```python
from build123d import *

# Parameters (mm, degrees)
SKETCH1_R           = 1.75
SKETCH1_W           = 15
SKETCH1_H           = 5
BOSS_EXTRUDE1_DEPTH = 5
FILLET1_R           = 5


with BuildPart() as part:
    # Sketch1 → Boss-Extrude1 (new body)
    with BuildSketch(Plane(origin=(0, 0, 0), x_dir=(1, 0, 0), z_dir=(0, 1, 0))):
        Polygon((65, 15), (65, 30), (60, 30), (60, 35), (50, 35), (50, 30), (0, 30), (0, 35), (-10, 35), (-10, 30), (-65, 30), (-65, 20), (-72.992352801, 20), (-72.992352801, 5), (-72.992352801, -5), (-72.992352801, -20), (-65, -20), (-65, -30), (-10, -30), (-10, -35), (0, -35), (0, -30), (50, -30), (50, -35), (60, -35), (60, -30), (65, -30), (65, -15), (85, -15), (85, -5), (65, -5), (65, 5), (85, 5), (85, 15), align=None)
        with Locations(Location((27, 20, 0), (0, 0, 270))):
            Circle(SKETCH1_R, mode=Mode.SUBTRACT)
        with Locations(Location((27, -20, 0), (0, 0, 270))):
            Circle(SKETCH1_R, mode=Mode.SUBTRACT)
        with Locations(Location((-31, 20.3, 0), (0, 0, 270))):
            Circle(SKETCH1_R, mode=Mode.SUBTRACT)
        with Locations(Location((-31, -20.3, 0), (0, 0, 270))):
            Circle(SKETCH1_R, mode=Mode.SUBTRACT)
        with Locations((72.5, 10)):
            Rectangle(SKETCH1_W, SKETCH1_H, mode=Mode.SUBTRACT)
        with Locations((72.5, -10)):
            Rectangle(SKETCH1_W, SKETCH1_H, mode=Mode.SUBTRACT)
        with Locations((-62.5, 12.5)):
            Rectangle(SKETCH1_W, SKETCH1_H, mode=Mode.SUBTRACT)
        with Locations((-62.5, -12.5)):
            Rectangle(SKETCH1_W, SKETCH1_H, mode=Mode.SUBTRACT)
    extrude(amount=BOSS_EXTRUDE1_DEPTH)

    # Fillet1
    fillet1_edges = [part.edges().sort_by_distance(p)[0] for p in [
        (65, 2.5, -15),
        (65, 2.5, -5),
        (65, 2.5, 5),
        (65, 2.5, 15),
    ]]
    fillet(fillet1_edges, radius=FILLET1_R - 0.0001)  # a hair under: the kernel refuses the full size


solid = part.part
```
For this review, take the finished solid that the model builds, in its own axes (mm). A direction names the side the tool comes from. Coordinates: 2 decimals unless noted, no trailing zeros. Loops run counter-clockwise (first coordinate to the right, second up) from the corner with the lowest first, then second, coordinate; pieces in that order, holes last.
1. Add section A-A, the plane x = 27. Give the boundary of the cut face in (y, z), then the cut area to 3 significant figures.
2. Insertion check: P1, Ø2.5, axis at x = 22, y = 2.5, coming from the +Z side; P2, Ø1.5, axis at y = 1.5, z = -27.5, coming from the -X side; P3, Ø1.5, axis at x = -70, y = 1.5, coming from the +Z side. Each pin has a flat end and moves straight along its axis. Give the tip position at first contact, or say it passes through.
3. Add section D-D, the plane x = -49. Give the boundary of the cut face in (y, z).
4. For line 1 (X direction, y = 1.1, z = -20.3); line 2 (X direction, y = 0.6, z = 8); line 3 (Z direction, x = -11, y = 0.8), list the stretches that pass through material, from the lowest coordinate up.
5. Add section B-B, the plane y = 1. Count the separate pieces of the cut face and the enclosed holes in it, then the cut area to 3 significant figures.
6. Mouldability with a two-part tool opening along X and no side actions: class faces 1 (the flat face through (-10, 2, 32)), 2 (the flat face through (55, 2, -35)), 3 (the cylindrical face through (-30.474, 2.465, 21.969)) as +X half, -X half, draft (parallel to the pull), parting line (faces both ways), or undercut.
7. For faces 4 (the flat face through (72, 2, 7.5)), 5 (the flat face through (0, 2, 33)), 6 (the flat face through (60, 2, 33)), 7 (the flat face through (77, 2, -5)), list the 3-axis set-ups (+Z, -Z, +X, -X, +Y, -Y) from which the entire face can be reached by the end or side of a thin tool; tool diameter is ignored.
8. Add section C-C, the plane z = -24. Give the boundary of the cut face in (x, y), then the cut area to 3 significant figures.
Result:
1. outline: (0, -30) - (5, -30) - (5, -21.75) - (0, -21.75) - close; (0, -18.25) - (5, -18.25) - (5, 18.25) - (0, 18.25) - close; (0, 21.75) - (5, 21.75) - (5, 30) - (0, 30) - close
1. area: 265 mm2
2. P1: stops at z = 30
2. P2: stops at x = -65
2. P3: stops at z = 20
3. outline: (0, -30) - (5, -30) - (5, 30) - (0, 30) - close
4. line 1: x = -65 to -32.75, -29.25 to 25.28, 28.72 to 65
4. line 2: x = -72.99 to 65, 80 to 85
4. line 3: z = -30 to 30
5. separate pieces: 1
5. enclosed holes: 8
5. area: 8,400 mm2
6. face 1: -X half
6. face 2: draft
6. face 3: undercut
7. face 4: +Y, -Y
7. face 5: +Z, +Y, -Y
7. face 6: +Z, +X, +Y, -Y
7. face 7: +X, +Y, -Y
8. outline: (-65, 0) - (65, 0) - (65, 5) - (-65, 5) - close
8. area: 650 mm2
